Part model, mm, in its own coordinate system. Give positions to 0.01 mm unless a question says otherwise; leave off trailing zeros. Write each loop counter-clockwise with the first axis right and the second up, starting at its lowest first coordinate (ties: lowest second). Pieces come first, ordered by that corner, then holes. Notation, with made-up numbers: M 47,46.5 L 74,46.5 A25 ccw 74,81.5 Z; hole C 34.5,2 d7. An arc over 180 degrees is marked long. Write item = value, one per line. Start each with the question number.
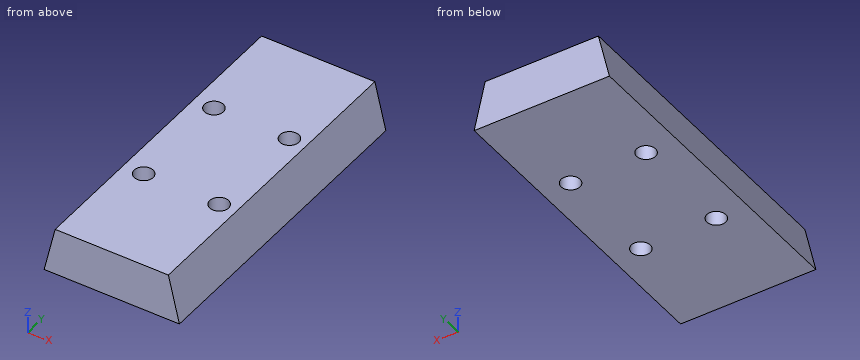
from build123d import *

# Parameters (mm, degrees)
CYLINDER001_R     = 3
CYLINDER001_DEPTH = 20
CYLINDER002_R     = 3
CYLINDER002_DEPTH = 20
CYLINDER003_R     = 3
CYLINDER003_DEPTH = 20
CYLINDER_R        = 3
CYLINDER_DEPTH    = 20
EXTRUDE_DEPTH     = 100


with BuildPart() as obj1:
    # Cylinder001 → Cylinder001 (new body)
    with BuildSketch(Plane(origin=(0, 34, 0), x_dir=(1, 0, 0), z_dir=(0, 0, 1))):
        Circle(CYLINDER001_R)
    extrude(amount=CYLINDER001_DEPTH)


with BuildPart() as obj2:
    # Cylinder002 → Cylinder002 (new body)
    with BuildSketch(Plane(origin=(24, 34, 0), x_dir=(1, 0, 0), z_dir=(0, 0, 1))):
        Circle(CYLINDER002_R)
    extrude(amount=CYLINDER002_DEPTH)


with BuildPart() as obj3:
    # Cylinder003 → Cylinder003 (new body)
    with BuildSketch(Plane(origin=(24, 0, 0), x_dir=(1, 0, 0), z_dir=(0, 0, 1))):
        Circle(CYLINDER003_R)
    extrude(amount=CYLINDER003_DEPTH)


with BuildPart() as fusion:
    # Cylinder → Cylinder (new body)
    with BuildSketch(Plane.XY):
        Circle(CYLINDER_R)
    extrude(amount=CYLINDER_DEPTH)

    # Fusion: union obj1, obj2, obj3
    add(obj1.part)
    add(obj2.part)
    add(obj3.part)


with BuildPart() as fusion_1:
    # Fusion placement: moved
    add(fusion.part.moved(Location((10, -67, 0))))


with BuildPart() as cut:
    # Sketch → Extrude (new body)
    with BuildSketch(Plane.XZ):
        Polygon((0, 0), (43, 0), (39.5, 15), (3.5, 15), align=None)
    extrude(amount=EXTRUDE_DEPTH)

    # Cut: cut Fusion
    add(fusion_1.part, mode=Mode.SUBTRACT)


solid = cut.part
Q1. Drop flat-ended pins along their axis: P1, Ø1.5, axis at y = -63.5, z = 10.5, coming from the +X side (3 decimals); P2, Ø3, axis at y = -89, z = 2.5, coming from the -X side; P3, Ø1, axis at x = 17, z = 5.5, coming from the +Y side; P4, Ø1, axis at x = 9.5, y = -33, coming from the +Z side. Give the stop position or say it passes through.
Q2. Slice it at C-C (z = 6.5). Give the cut face in (x, y).
Q3. Probe line 1 along Y through (x, z) = (34, 10.75); line 2 along Y through (x, z) = (9, 1); line 3 along X through (y, z) = (-33, 8.5). List the from-to ranges inside material, lowest first.
Q4. Slice it at A-A (y = -33). Give the cut face in (x, z), and give its area (4 significant figures).
Q5. Slice it at B-B (x = 34). Give the cut face in (y, z), and give its area (3 significant figures).
Q6. Slice it at D-D (y = -16). Give the cut face in (x, z).
Working result:
q1.P1 = 40.725
q1.P2 = 0.23
q1.P3 = 0
q1.P4 = through
q2.outline = M 1.52,-100 L 41.48,-100 L 41.48,0 L 1.52,0 Z; hole C 10,-67 d6; hole C 10,-33 d6; hole C 34,-67 d6; hole C 34,-33 d6
q3.line_1 = -100 to -70, -64 to -36, -30 to 0
q3.line_2 = -100 to -69.83, -64.17 to -35.83, -30.17 to 0
q3.line_3 = 1.98 to 7, 13 to 31, 37 to 41.02
q4.outline = M 0,0 L 7,0 L 7,15 L 3.5,15 Z; M 13,0 L 31,0 L 31,15 L 13,15 Z; M 37,0 L 43,0 L 39.5,15 L 37,15 Z
q4.area = 412.5 mm2
q5.outline = M -100,0 L -70,0 L -70,15 L -100,15 Z; M -64,0 L -36,0 L -36,15 L -64,15 Z; M -30,0 L 0,0 L 0,15 L -30,15 Z
q5.area = 1,320 mm2
q6.outline = M 0,0 L 43,0 L 39.5,15 L 3.5,15 Z
